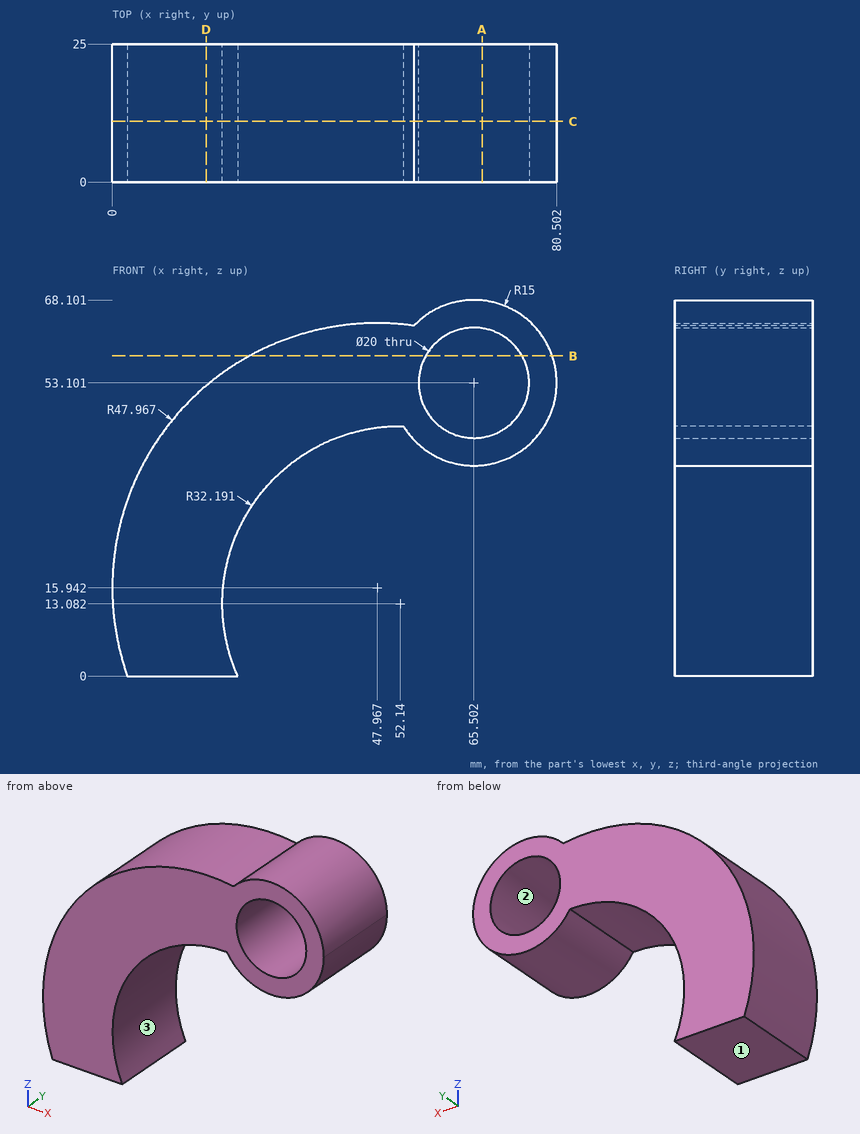
Check sheet for the drawn part. Datum: minimum x, y, z corner. Units: mm. Give positions to 0.01 mm unless a question says otherwise; leave off trailing zeros. Write each loop counter-clockwise with the first axis right and the second up, starting at its lowest first coordinate (ties: lowest second). Pieces come first, ordered by that corner, then holes. Notation, with made-up numbers: (-11.75, 72.25) -> (45.25, 72.25) arc R15 ccw to (45.25, 98.25) -> close; hole circle Ø11 at (61.5, 27.25). An arc over 180 degrees is marked (long way). Use one line per item in the form item = value. Start each with the question number.
1. Go/stop test with flat-tipped pins: P1, Ø3, axis at y = 7.5, z = 47.5, coming from the +X side; P2, Ø10, axis at x = 50.5, y = 9.5, coming from the -Z side; P3, Ø8, axis at x = 26.5, z = 55.5, coming from the -Y side; P4, Ø12, axis at y = 17, z = 33.5, coming from the +X side (1 decimal). Record where each tip stops, or that it passes through.
2. Section check C-C (y = 11). Record the cut outline in (x, z) (1 decimal).
3. Section check B-B (z = 58). Record the cut outline in (x, y) (1 decimal).
4. Mould release check, pull along X, two halves, no side actions. Record for the marked faces 1, 2 and 3: pulls with the +X half, pulls with the -X half, needs draft (parallel to the pull), parting line crosses it, or undercut.
5. Section check D-D (x = 17). Record the cut outline in (y, z).
6. Section check A-A (x = 67). Record the cut outline in (y, z) (1 decimal).
7. Thickness scan on line 1 along Z through (x, y) = (57, 10.5) (1 decimal); line 2 along X through (y, z) = (12.25, 50.5) (1 decimal); line 3 along X through (y, z) = (14.25, 46) (1 decimal). Record the ranges inside material, lowest first. Write a range as from..to.
Conclusion:
q1.P1 = 79.93
q1.P2 = 41.92
q1.P3 = 0
q1.P4 = 71.8
q2.outline = (2.7, 0) -> (22.7, 0) arc R32.2 cw to (52.7, 45.3) arc R15 ccw (long way) to (54.6, 63.4) arc R48 ccw to start; hole circle Ø20 at (65.5, 53.1)
q3.outline = (24.9, 0) -> (56.8, 0) -> (56.8, 25) -> (24.9, 25) -> close; (74.2, 0) -> (79.7, 0) -> (79.7, 25) -> (74.2, 25) -> close
q4.face_1 = needs draft
q4.face_2 = undercut
q4.face_3 = undercut
q5.outline = (0, 0) -> (25, 0) -> (25, 52.57) -> (0, 52.57) -> close
q6.outline = (0, 38.2) -> (25, 38.2) -> (25, 43.2) -> (0, 43.2) -> close; (0, 63) -> (25, 63) -> (25, 68) -> (0, 68) -> close
q7.line_1 = 40.7..47.8, 58.4..65.5
q7.line_2 = 14.7..55.8, 75.2..80.3
q7.line_3 = 10.6..58.5, 72.5..78.7
